Can you work these out from the model? Positions are in its coordinate system, mm. A direction names the side the tool comes from. Round coordinates to 2 decimals unless told otherwise and drop trailing zeros. Order: outer loops, then holes, each group sorted by start corner. A loop starts at its lowest first (then second) coordinate and runs counter-clockwise, first axis right, second up. Notation, with made-up numbers: M 15,59.5 L 52,59.5 A9 ccw 52,75.5 Z; hole C -29.5,49 d11. An arc over 180 degrees is marked long. One line per question, with ' | ' between items.
```python
from build123d import *

# Parameters (mm, degrees)
SKETCH2_W           = 59
SKETCH2_H           = 31
BOSS_EXTRUDE1_DEPTH = 21.5
SKETCH3_W           = 8.3
SKETCH3_H           = 8.3
SKETCH3_R           = 1.95
BOSS_EXTRUDE2_DEPTH = 2.71


with BuildPart() as part:
    # Sketch2 → Boss-Extrude1 (new body)
    with BuildSketch(Plane(origin=(0, 0, 0), x_dir=(1, 0, 0), z_dir=(0, 1, 0))):
        Rectangle(SKETCH2_W, SKETCH2_H)
    extrude(amount=BOSS_EXTRUDE1_DEPTH)

    # Sketch3 → Boss-Extrude2 (add)
    # profile 1 of 2: a face of its own
    with BuildSketch(Plane.XZ):
        with Locations((-33.65, 0)):
            Rectangle(SKETCH3_W, SKETCH3_H)
        with Locations(Location((-33.25, 0, 0), (0, 0, 270))):
            Circle(SKETCH3_R, mode=Mode.SUBTRACT)
    # profile 2 of 2: a face of its own
    with BuildSketch(Plane.XZ):
        with Locations((33.65, 0)):
            Rectangle(SKETCH3_W, SKETCH3_H)
        with Locations(Location((33.25, 0, 0), (0, 0, 90))):
            Circle(SKETCH3_R, mode=Mode.SUBTRACT)
    extrude(amount=-BOSS_EXTRUDE2_DEPTH)


solid = part.part
```
(1) Will these pins go through, and if not, where does the flat tip stop? pin 1 Ø0.8 at (x, y) = (32, 1) entering from -Z; pin 2 Ø11 at (y, z) = (8, 5) entering from +X; pin 3 Ø4 at (x, z) = (32.5, -0.5) entering from +Y; pin 4 Ø6 at (y, z) = (11.5, -3) entering from +X.
Final values:
pin 1: z = -4.15 | pin 2: x = 37.8 | pin 3: y = 2.71 | pin 4: x = 29.5
(2) If we section it at B-B on z = 0: Please give me the cut outline in (x, y).
Final values:
outline: M -37.8,0 L -35.2,0 L -35.2,2.71 L -37.8,2.71 Z; M -31.3,0 L 31.3,0 L 31.3,2.71 L 29.5,2.71 L 29.5,21.5 L -29.5,21.5 L -29.5,2.71 L -31.3,2.71 Z; M 35.2,0 L 37.8,0 L 37.8,2.71 L 35.2,2.71 Z
(3) Please list where these lines run through material, in increasing order: probe 1 along X at (y, z) = (0.9, 0); probe 2 along Z at (x, y) = (33.25, 2.25); probe 3 along X at (y, z) = (3.25, 1). Write a range as [from, to].
Final values:
probe 1: [-37.8, -35.2], [-31.3, 31.3], [35.2, 37.8] | probe 2: [-4.15, -1.95], [1.95, 4.15] | probe 3: [-29.5, 29.5]
(4) On a 3-axis mill with a long thin cutter (end or side, diameter ignored), from which of +Z, -Z, +X, -X, +Y, -Y can I reach the whole of each face in a straight line? I mean faces 4 (the flat face through (34, 1, -4.15)), 5 (the flat face through (-34, 1, -4.15)), 6 (the flat face through (34, 1, 4.15)). Say none if no direction works.
Final values:
face 4: -Z, +X, +Y, -Y | face 5: -Z, -X, +Y, -Y | face 6: +Z, +X, +Y, -Y
(5) If we section it at C-C on y = 20: Please give me the cut outline in (x, z).
Final values:
outline: M -29.5,-15.5 L 29.5,-15.5 L 29.5,15.5 L -29.5,15.5 Z
(6) If we section it at A-A on x = -33.25: Please give me the cut outline in (y, z), plus the area to 3 significant figures.
Final values:
outline: M 0,-4.15 L 2.71,-4.15 L 2.71,-1.95 L 0,-1.95 Z; M 0,1.95 L 2.71,1.95 L 2.71,4.15 L 0,4.15 Z | area: 11.9 mm^2
(7) If we section it at D-D on z = -11.5: Please give me the cut outline in (x, y), plus the area to 3 significant figures.
Final values:
outline: M -29.5,0 L 29.5,0 L 29.5,21.5 L -29.5,21.5 Z | area: 1,270 mm^2
(8) Thinking about a two-plate mould opening in X: for faces 1 (the flat face through (-1, 0, 0)), 2 (the cylindrical face through (31.317, 1.336, -0.254)), 3 (the flat face through (-37.8, 1, 0)), which applies, released by +X, released by -X, zero draft, split by the parting line, or undercut?
Final values:
face 1: zero draft | face 2: undercut | face 3: released by -X
